Job drawing, mm, ordinate dimensions from the low corner. One solid piece. A direction names the side the tool comes from. Give positions to 0.01 mm unless a question says otherwise; leave off trailing zeros. Loops run counter-clockwise (first coordinate to the right, second up) from the corner with the lowest first, then second, coordinate; pieces in that order, holes last. Notation, with made-up numbers: M -17,59.25 L 26,59.25 A8 cw 26,68.25 Z; hole C 21.5,65 d7. An arc over 180 degrees is marked long. Put each result on its own line as item: value.
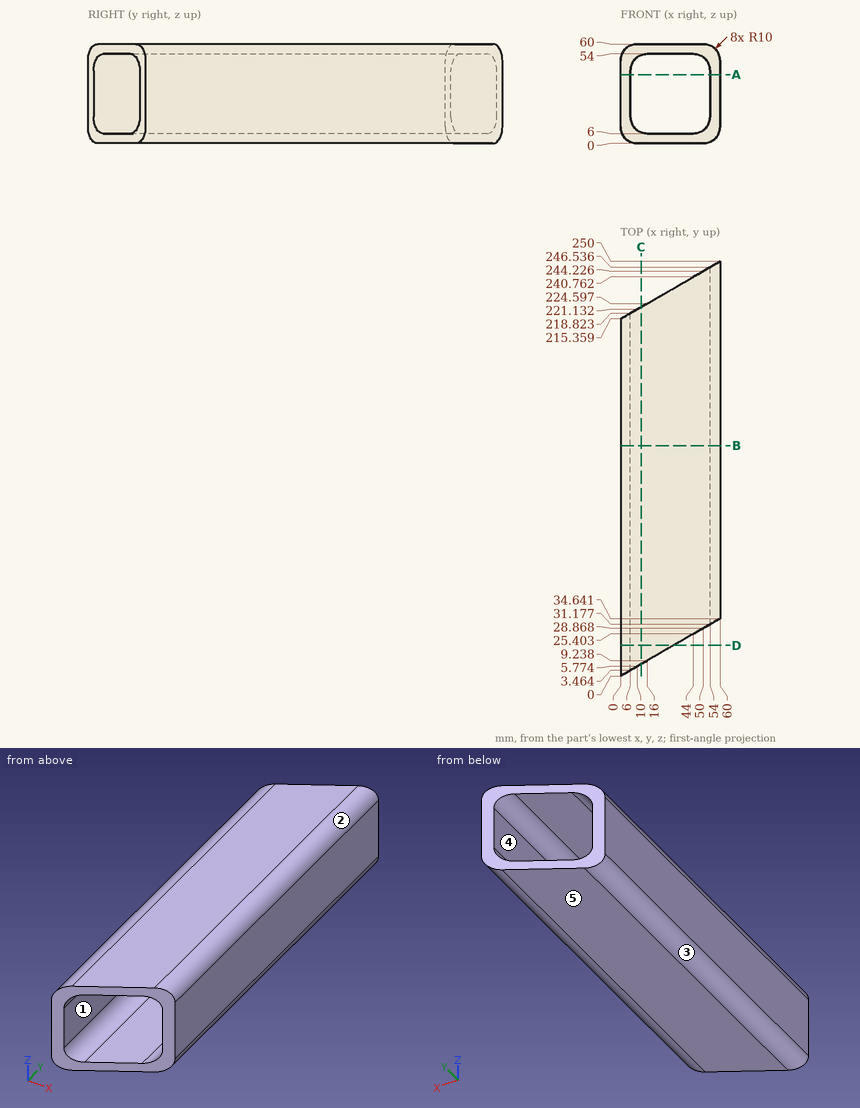
Q1. Mould opens along Z. For the marked faces 1, 2 and 3 say: pulls with the +Z half, pulls with the -Z half, needs draft (parallel to the pull), parting line crosses it, or undercut.
Here are the results:
face 1: undercut
face 2: pulls with the +Z half
face 3: pulls with the -Z half
Q2. Slice it at A-A (z = 41.5). List the corners of the cut face in (x, y) (1 decimal).
Here are the results:
outline: M 0,0 L 6,3.5 L 6,218.8 L 0,215.4 Z; M 54,31.2 L 60,34.6 L 60,250 L 54,246.5 Z
Q3. Probe line 1 (X direction, y = 208, z = 39); line 2 (Y direction, x = 50, z = 5.5) (1 decimal). List the from-to ranges inside material, lowest first. Write a range as from..to.
Here are the results:
line 1: 0..6, 54..60
line 2: 28.9..244.2
Q4. Drop flat-ended pins along their axis: pin 1 Ø22.5 at (y, z) = (96.5, 28) entering from -X; pin 2 Ø2 at (x, z) = (51.5, 52.5) entering from -Y (1 decimal); pin 3 Ø4 at (y, z) = (207, 6.5) entering from +X. Give the stop position or say it passes through.
Here are the results:
pin 1: x = 0
pin 2: y = 29.2
pin 3: x = 59.89
Q5. Tool access for the marked faces 4 and 5: list every direction of +Z, -Z, +X, -X, +Y, -Y with a clear straight run to the whole face (end or side of a thin tool).
Here are the results:
face 4: +Y, -Y
face 5: -Z, +X, -X, +Y, -Y
Q6. Slice it at C-C (x = 12.5). List the corners of the cut face in (y, z) (1 decimal).
Here are the results:
outline: M 7.2,0 L 222.6,0 L 222.6,6.6 L 7.2,6.6 Z; M 7.2,53.4 L 222.6,53.4 L 222.6,60 L 7.2,60 Z
Q7. Slice it at D-D (y = 18.5). List the corners of the cut face in (x, z).
Here are the results:
outline: M 0,10 A10 ccw 10,0 L 32.04,0 L 32.04,6 L 16,6 A10 cw 6,16 L 6,44 A10 cw 16,54 L 32.04,54 L 32.04,60 L 10,60 A10 ccw 0,50 Z
Q8. Slice it at B-B (y = 139). List the corners of the cut face in (x, z), and give its area (3 significant figures).
Here are the results:
outline: M 0,10 A10 ccw 10,0 L 50,0 A10 ccw 60,10 L 60,50 A10 ccw 50,60 L 10,60 A10 ccw 0,50 Z; hole M 6,16 A10 ccw 16,6 L 44,6 A10 ccw 54,16 L 54,44 A10 ccw 44,54 L 16,54 A10 ccw 6,44 Z
area: 1,300 mm²
